Geometry check sheet. Reference: the model listing, model coordinates, mm. A direction names the side the tool comes from. Coordinates: 2 decimals unless noted, no trailing zeros. Write each loop counter-clockwise with the first axis right and the second up, starting at its lowest first coordinate (ties: lowest second). Pieces come first, ordered by that corner, then holes.
from build123d import *

# Parameters (mm, degrees)
F1_DEPTH = 320
F2_R     = 5
F3_DEPTH = 1.2
F4_R     = 5
F6_DEPTH = 1.2
F7_R     = 2.5
F8_DEPTH = 2


with BuildPart() as f1:
    # F0 (on Front) → F1 (new body)
    with BuildSketch(Plane.XZ):
        with BuildLine():
            Line((1.2, 0), (0, 0))
            Line((0, 0), (0, -167))
            ThreePointArc((0, -167), (-1.464466, -170.535534), (-5, -172))
            Line((-5, -172), (-30, -172))
            Line((-30, -172), (-30, -173.2))
            Line((-30, -173.2), (-5, -173.2))
            ThreePointArc((-5, -173.2), (-0.615938, -171.384062), (1.2, -167))
            Line((1.2, -167), (1.2, 0))
        make_face()
    extrude(amount=-F1_DEPTH)

    # F2 (on face) → F3 (cut, through all)
    with BuildSketch(Plane.XY.offset(-172)):
        with Locations((-17.5, 305)):
            Circle(F2_R)
        with Locations((-17.5, 15)):
            Circle(F2_R)
    extrude(amount=-F3_DEPTH, mode=Mode.SUBTRACT)

    # F4
    f4_edges = [f1.edges().sort_by_distance(p)[0] for p in [
        (-30, 320, -172.6),
        (-30, 0, -172.6),
    ]]
    fillet(f4_edges, radius=F4_R)

    # F5 (on face) → F6 (cut, through all)
    with BuildSketch(Plane(origin=(0, 0, 0), x_dir=(0, -1, 0), z_dir=(-1, 0, 0))):
        Polygon((0, 0), (-320, 0), (0, -10), align=None)
    extrude(amount=-F6_DEPTH, mode=Mode.SUBTRACT)

    # F7 (on face) → F8 (cut)
    with BuildSketch(Plane.YZ.offset(1.2)):
        with Locations((10, -30)):
            Circle(F7_R)
        with Locations((159.926811, -25.314787)):
            Circle(F7_R)
        with Locations((309.853623, -20.629574)):
            Circle(F7_R)
    extrude(amount=-F8_DEPTH, mode=Mode.SUBTRACT)


solid = f1.part
1. Sectioned sample at A-A, the plane x = -17.5. Record the boundary of the cut face in (y, z), and give its area (3 significant figures).
Computed values:
outline: (0, -173.2) - (10, -173.2) - (10, -172) - (0, -172) - close; (20, -173.2) - (300, -173.2) - (300, -172) - (20, -172) - close; (310, -173.2) - (320, -173.2) - (320, -172) - (310, -172) - close
area: 360 mm2
2. Gauge pin test, flat ends, axial feed: pin 1 Ø5 at (x, y) = (-22, 161) entering from +Z; pin 2 Ø1 at (y, z) = (222, -105) entering from -X; pin 3 Ø3 at (y, z) = (309.85, -20.63) entering from +X. Record the tip position at first contact, or that the pin passes through.
Computed values:
pin 1: stops at z = -172
pin 2: stops at x = 0
pin 3: passes through
3. Access from +Z, -Z, +X, -X, +Y, -Y to the whole of each face (thin tool, end or side, straight path). Record for faces 4 (the cylindrical face through (-18.151, 309.957, -172.592)), 5 (the flat face through (-17, 158, -172)).
Computed values:
face 4: +Z, -Z
face 5: +Z, -X, +Y, -Y
4. Sectioned sample at D-D, the plane y = 255. Record the boundary of the cut face in (x, z).
Computed values:
outline: (-30, -173.2) - (-5, -173.2) arc R6.2 ccw to (1.2, -167) - (1.2, -2.03) - (0, -2.03) - (0, -167) arc R5 cw to (-5, -172) - (-30, -172) - close
5. Sectioned sample at B-B, the plane y = 85.5. Record the boundary of the cut face in (x, z).
Computed values:
outline: (-30, -173.2) - (-5, -173.2) arc R6.2 ccw to (1.2, -167) - (1.2, -7.33) - (0, -7.33) - (0, -167) arc R5 cw to (-5, -172) - (-30, -172) - close
6. Sectioned sample at C-C, the plane z = -115.5. Record the boundary of the cut face in (x, y).
Computed values:
outline: (0, 0) - (1.2, 0) - (1.2, 320) - (0, 320) - close
7. Draft check along Y on faces 1 (the cylindrical face through (-0.66, 157.76, -171.43)), 2 (the flat face through (1, 0, -91)), 3 (the cylindrical face through (-18.58, 10.12, -172.59)). Enter one of: released by +Y, released by -Y, zero draft, split by the parting line, or undercut.
Computed values:
face 1: zero draft
face 2: released by -Y
face 3: undercut
8. Thickness scan on line 1 along Y through (x, z) = (-17.5, -172.8); line 2 along Z through (x, y) = (-4.5, 118.5); line 3 along X through (y, z) = (117, -18.5). Record the ranges inside material, lowest first.
Computed values:
line 1: y = 0 to 10, 20 to 300, 310 to 320
line 2: z = -173.18 to -171.97
line 3: x = 0 to 1.2
